Model file for the job. Use its own axes, mm. Face numbers are marked on the shaded views. Give positions to 0.01 mm unless a question says otherwise; leave off trailing zeros. Order: outer loops, then holes, each group sorted by start corner. A loop starts at its lowest first (then second) coordinate and runs counter-clockwise, first axis right, second up. Notation, with made-up numbers: M 40,-2.75 L 62,-2.75 A21 ccw 62,4.25 Z; hole C 85.25,-20.75 d7. An arc over 180 degrees is marked long. Return JSON: item names as keys, results as strings. Group by question number.
1. Wall check: probe 1 along X at (y, z) = (70.5, 176); probe 2 along Y at (x, z) = (118.5, 146.5); probe 3 along Y at (x, z) = (237, 42). Give the ranges that are in metal, low to high. Write a range as [from, to].
2. Two-plate mould, pull along X, no slides. Class the marked faces 1, 2, 3 and 4: released by +X, released by -X, zero draft, split by the parting line, or undercut.
3. Pin check, flat tips, straight feed: pin 1 (7.5 mm diameter, centred on x = 119, y = 78, fed in from +Z); pin 2 (8 mm diameter, centred on x = 172, z = 125, fed in from -Y); pin 3 (1.6 mm diameter, centred on y = 77.66, z = 140.64, fed in from -X); pin 4 (12 mm diameter, centred on x = 254.5, y = 84.5, fed in from +Z). Stop position of each tip, or through.
4. Slice it at D-D on x = 82. List the corners of the cut face in (y, z), then the cut area to 3 significant figures.
5. Slice it at C-C on z = 52.5. List the corners of the cut face in (x, y), then the cut area to 3 significant figures.
6. Slice it at A-A on y = 214. List the corners of the cut face in (x, z).
7. Slice it at B-B on x = 18.5. List the corners of the cut face in (y, z).
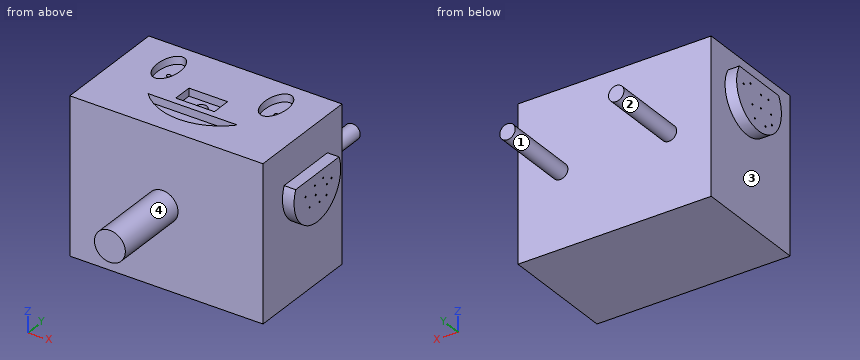
Autodesk Inventor part; units mm, degrees
ref_plane "YZ Plane" through (0, 0, 0) normal (1, 0, 0) x (0, 1, 0)
ref_plane "XZ Plane" through (0, 0, 0) normal (0, 1, 0) x (-1, 0, 0)
ref_plane "XY Plane" through (0, 0, 0) normal (0, 0, 1) x (1, 0, 0)
sketch "Sketch1" plane through (0, 0, 0) normal (0, 0, 1) x (1, 0, 0)
  line L0 (0, 0) -> (250, 0)
  line L1 (250, 0) -> (250, 150)
  line L2 (250, 150) -> (0, 150)
  line L3 (0, 150) -> (0, 0)
  ellipse E0 centre (61.2005, 103.0437) end of major axis (61.2005, 79.9077) minor radius 20.4496
  ellipse E1 centre (186.6962, 103.0437) end of major axis (186.6962, 79.9077) minor radius 20.4496
  arc A0 (59.086, 49.2762) -> (190.914, 49.2762) centre (125, 119.8778) ccw
  line L4 (59.086, 49.2762) -> (190.914, 49.2762)
extrude "Extrusion1" add sketch "Sketch1" along normal blind 200 contours L3 L2 L1 L0 | E0 | E1 | L4 A0
sketch "Sketch2" plane through (0, 0, 0) normal (0, 0, -1) x (-1, 0, 0)
  point P0 (0, 0)
sketch "Sketch3" plane through (0, 0, 200) normal (0, 0, 1) x (1, 0, 0)
  ellipse E0 centre (54.3866, 108.1481) end of major axis (54.3866, 81.8925) minor radius 14.5317
  ellipse E1 centre (193.1662, 108.1481) end of major axis (193.1662, 81.8925) minor radius 14.5317
  arc A0 (66.4831, 50.9455) -> (182.3199, 50.9455) centre (124.4015, 103.7721) ccw
  line L0 (66.4831, 50.9455) -> (182.3199, 50.9455)
  point P0 (0, 0)
extrude "Extrusion2" cut sketch "Sketch3" against normal blind 10 contours E0
extrude "Extrusion3" cut sketch "Sketch3" against normal blind 10 contours E1
extrude "Extrusion4" cut sketch "Sketch3" against normal blind 10 contours L0 A0
sketch "Sketch4" plane through (250, 0, 0) normal (1, 0, 0) x (0, 0, -1)
  arc A0 (-152.7748, 40.0737) -> (-152.7748, 122.4086) centre (-136.5666, 81.2411) ccw
  line L0 (-152.7748, 40.0737) -> (-152.7748, 122.4086)
  point P0 (0, 0)
extrude "Extrusion5" add sketch "Sketch4" along normal blind 15
sketch "Sketch5" plane through (0, 0, 0) normal (-1, 0, 0) x (0, 0, 1)
  line L0 (152.7748, 40.0737) -> (152.7748, 122.4086)
  arc A0 (173.1982, 118.4375) -> (173.1982, 44.0448) centre (152.7748, 81.2411) ccw
  line L1 (173.1982, 118.4375) -> (173.1982, 44.0448)
  point P0 (0, 0)
extrude "Extrusion6" add sketch "Sketch5" along normal blind 15
sketch "Sketch6" plane through (0, 150, 0) normal (0, 1, 0) x (1, 0, 0)
  circle A0 centre (54.7125, -97.0495) radius 10
  circle A1 centre (195.4016, -97.0495) radius 10
  point P0 (0, 0)
  dimension "d14" = 20
  dimension "d15" = 20
extrude "Extrusion7" add sketch "Sketch6" along normal blind 100 contours A0
extrude "Extrusion8" add sketch "Sketch6" along normal blind 100 contours A1
sketch "Sketch7" plane through (0, 0, 0) normal (0, -1, 0) x (1, 0, 0)
  point P0 (0, 0)
sketch "Sketch9" plane through (0, 0, 0) normal (0, -1, 0) x (1, 0, 0)
  circle A0 centre (120.0971, 102.6638) radius 20
  point P0 (0, 0)
  dimension "d20" = 40
extrude "Extrusion9" add sketch "Sketch9" along normal blind 100
sketch "Sketch10" plane through (-15, 0, 0) normal (-1, 0, 0) x (0, 0, 1)
  point P0 (0, 0)
  point P1 (140.6371, 77.6587)
hole "Hole1" at (-15, 77.6587, 140.6371) direction (1, 0, 0) diameter 2 depth 5 tip angle 118
sketch "Sketch11" plane through (-15, 0, 0) normal (-1, 0, 0) x (0, 0, 1)
  point P0 (0, 0)
  point P1 (137.5819, 94.0305)
hole "Hole2" at (-15, 94.0305, 137.5819) direction (1, 0, 0) diameter 2 depth 5 tip angle 118
sketch "Sketch12" plane through (-15, 0, 0) normal (-1, 0, 0) x (0, 0, 1)
  point P0 (0, 0)
  point P1 (161.7546, 97.274)
hole "Hole3" at (-15, 97.274, 161.7546) direction (1, 0, 0) diameter 2 depth 5 tip angle 118
sketch "Sketch13" plane through (-15, 0, 0) normal (-1, 0, 0) x (0, 0, 1)
  point P0 (0, 0)
  point P1 (122.1615, 69.1759)
hole "Hole4" at (-15, 69.1759, 122.1615) direction (1, 0, 0) diameter 2 depth 5 tip angle 118
sketch "Sketch14" plane through (-15, 0, 0) normal (-1, 0, 0) x (0, 0, 1)
  point P0 (0, 0)
  point P1 (142.1664, 58.2443)
hole "Hole5" at (-15, 58.2443, 142.1664) direction (1, 0, 0) diameter 2 depth 5 tip angle 118
sketch "Sketch15" plane through (-15, 0, 0) normal (-1, 0, 0) x (0, 0, 1)
  point P0 (0, 0)
  point P1 (154.8779, 110.2581)
hole "Hole6" at (-15, 110.2581, 154.8779) direction (1, 0, 0) diameter 2 depth 5 tip angle 118
sketch "Sketch16" plane through (-15, 0, 0) normal (-1, 0, 0) x (0, 0, 1)
  point P0 (0, 0)
  point P1 (158.2121, 63.5601)
hole "Hole7" at (-15, 63.5601, 158.2121) direction (1, 0, 0) diameter 2 depth 5 tip angle 118
sketch "Sketch17" plane through (-15, 0, 0) normal (-1, 0, 0) x (0, 0, 1)
  point P0 (0, 0)
  point P1 (157.5869, 77.3239)
hole "Hole8" at (-15, 77.3239, 157.5869) direction (1, 0, 0) diameter 2 depth 5 tip angle 118
sketch "Sketch18" plane through (-15, 0, 0) normal (-1, 0, 0) x (0, 0, 1)
  point P0 (0, 0)
  point P1 (122.5782, 89.2357)
hole "Hole9" at (-15, 89.2357, 122.5782) direction (1, 0, 0) diameter 2 depth 5 tip angle 118
sketch "Sketch19" plane through (-15, 0, 0) normal (-1, 0, 0) x (0, 0, 1)
  point P0 (0, 0)
  point P1 (130.0801, 56.8932)
hole "Hole10" at (-15, 56.8932, 130.0801) direction (1, 0, 0) diameter 2 depth 5 tip angle 118
sketch "Sketch20" plane through (265, 0, 0) normal (1, 0, 0) x (0, 0, -1)
  point P0 (0, 0)
  point P1 (-130.0065, 99.3663)
hole "Hole11" at (265, 99.3663, 130.0065) direction (-1, 0, 0) diameter 2 depth 5 tip angle 118
sketch "Sketch21" plane through (265, 0, 0) normal (1, 0, 0) x (0, 0, -1)
  point P0 (0, 0)
  point P1 (-115.2751, 85.4238)
hole "Hole12" at (265, 85.4238, 115.2751) direction (-1, 0, 0) diameter 2 depth 5 tip angle 118
sketch "Sketch22" plane through (265, 0, 0) normal (1, 0, 0) x (0, 0, -1)
  point P0 (0, 0)
  point P1 (-139.5268, 76.7471)
hole "Hole13" at (265, 76.7471, 139.5268) direction (-1, 0, 0) diameter 2 depth 5 tip angle 118
sketch "Sketch23" plane through (265, 0, 0) normal (1, 0, 0) x (0, 0, -1)
  point P0 (0, 0)
  point P1 (-117.355, 66.6893)
hole "Hole14" at (265, 66.6893, 117.355) direction (-1, 0, 0) diameter 2 depth 5 tip angle 118
sketch "Sketch24" plane through (265, 0, 0) normal (1, 0, 0) x (0, 0, -1)
  point P0 (0, 0)
  point P1 (-117.0358, 98.3789)
hole "Hole15" at (265, 98.3789, 117.0358) direction (-1, 0, 0) diameter 2 depth 5 tip angle 118
sketch "Sketch25" plane through (265, 0, 0) normal (1, 0, 0) x (0, 0, -1)
  point P0 (0, 0)
  point P1 (-134.2147, 59.0465)
hole "Hole16" at (265, 59.0465, 134.2147) direction (-1, 0, 0) diameter 2 depth 5 tip angle 118
sketch "Sketch26" plane through (265, 0, 0) normal (1, 0, 0) x (0, 0, -1)
  point P0 (0, 0)
  point P1 (-127.1753, 78.1775)
hole "Hole17" at (265, 78.1775, 127.1753) direction (-1, 0, 0) diameter 2 depth 5 tip angle 118
sketch "Sketch27" plane through (265, 0, 0) normal (1, 0, 0) x (0, 0, -1)
  point P0 (0, 0)
  point P1 (-141.5728, 92.3364)
hole "Hole18" at (265, 92.3364, 141.5728) direction (-1, 0, 0) diameter 2 depth 5 tip angle 118
sketch "Sketch28" plane through (265, 0, 0) normal (1, 0, 0) x (0, 0, -1)
  point P0 (0, 0)
  point P1 (-133.6045, 107.8408)
hole "Hole19" at (265, 107.8408, 133.6045) direction (-1, 0, 0) diameter 2 depth 5 tip angle 118
sketch "Sketch29" plane through (0, 0, 200) normal (0, 0, 1) x (1, 0, 0)
  line L0 (96.2975, 84.9409) -> (146.2975, 84.9409)
  line L1 (146.2975, 84.9409) -> (146.2975, 59.9409)
  line L2 (146.2975, 59.9409) -> (96.2975, 59.9409)
  line L3 (96.2975, 59.9409) -> (96.2975, 84.9409)
  point P0 (0, 0)
  dimension "d156" = 50
  dimension "d157" = 25
extrude "Extrusion10" cut sketch "Sketch29" against normal blind 10
sketch "Sketch30" plane through (0, 0, 190) normal (0, 0, 1) x (1, 0, 0)
  circle A0 centre (121.2975, 71.6727) radius 7.5
  point P0 (0, 0)
  dimension "d160" = 15
extrude "Extrusion11" cut sketch "Sketch30" against normal blind 50
sketch "Sketch31" plane through (0, 0, 190) normal (0, 0, 1) x (1, 0, 0)
  point P0 (0, 0)
  point P1 (54.4067, 107.7576)
hole "Hole20" at (54.4067, 107.7576, 190) direction (0, 0, -1) diameter 5 depth 5 tip angle 118
sketch "Sketch32" plane through (0, 0, 190) normal (0, 0, 1) x (1, 0, 0)
  point P0 (0, 0)
  point P1 (195.0454, 105.5749)
hole "Hole21" at (195.0454, 105.5749, 190) direction (0, 0, -1) diameter 5 depth 5 tip angle 118
properties part number "head part 2"
Result:
{
 "1": {"probe 1": "x = [0, 113.89], [128.71, 250]", "probe 2": "y = [0, 64.71], [78.63, 150]", "probe 3": "y = [0, 150]"},
 "2": {"face 1": "undercut", "face 2": "undercut", "face 3": "released by -X", "face 4": "split by the parting line"},
 "3": {"pin 1": "stops at z = 190", "pin 2": "stops at y = 0", "pin 3": "stops at x = -9.88", "pin 4": "stops at z = 200"},
 "4": {"outline": "M 0,0 L 150,0 L 150,200 L 50.95,200 L 50.95,190 L 37.84,190 L 37.84,200 L 0,200 Z", "area": "29,900 mm2"},
 "5": {"outline": "M 0,0 L 250,0 L 250,150 L 0,150 Z", "area": "37,500 mm2"},
 "6": {"outline": "C 54.71,97.05 d20; C 195.4,97.05 d20"},
 "7": {"outline": "M 0,0 L 150,0 L 150,200 L 0,200 Z"}
}
